Can you work these out from the model? Positions are in its coordinate system, mm. Give positions to 0.01 mm unless a question says otherwise; leave off trailing zeros. Order: outer loops, then holes, each group sorted by start corner. A loop starts at its lowest first (then second) coordinate and runs counter-clockwise, first axis right, second up. Notation, with made-up numbers: M 54,51 L 74,51 A32 ccw 74,79 Z; hole C 2.5,17.5 d6. An arc over 180 degrees is marked long. Answer as a JSON object with one key per item and string values.
```python
from build123d import *

# Parameters (mm, degrees)
EXTRUDE_1_DEPTH     = 8
SKETCH_3_R          = 3.1
SKETCH_3_R_2        = 1.6
CUT_EXTRUDE_1_DEPTH = 65.237839316
SKETCH_4_R          = 6.1
CUT_EXTRUDE_2_DEPTH = 65.237839316


with BuildPart() as part:
    # 草图1 → 凸台-拉伸1 (new body)
    with BuildSketch(Plane(origin=(0, 0, 0), x_dir=(1, 0, 0), z_dir=(0, 1, 0))):
        with BuildLine():
            Line((-50, -12.5), (50, -12.5))
            ThreePointArc((50, -12.5), (62.5, 0), (50, 12.5))
            Line((50, 12.5), (-50, 12.5))
            ThreePointArc((-50, 12.5), (-62.5, 0), (-50, -12.5))
        make_face()
    extrude(amount=EXTRUDE_1_DEPTH)

    # 草图3 → 切除-拉伸1 (cut, through all)
    with BuildSketch(Plane(origin=(0, 8, 0), x_dir=(1, 0, 0), z_dir=(0, 1, 0))):
        with Locations(Location((-50, 0, 0), (0, 0, 270))):
            Circle(SKETCH_3_R)
        with Locations(Location((50, 8, 0), (0, 0, 270))):
            Circle(SKETCH_3_R_2)
        with Locations(Location((58, 0, 0), (0, 0, 270))):
            Circle(SKETCH_3_R_2)
        with Locations(Location((50, -8, 0), (0, 0, 270))):
            Circle(SKETCH_3_R_2)
        with Locations(Location((42, 0, 0), (0, 0, 270))):
            Circle(SKETCH_3_R_2)
        with Locations(Location((50, 0, 0), (0, 0, 270))):
            Circle(SKETCH_3_R)
    extrude(amount=-CUT_EXTRUDE_1_DEPTH, mode=Mode.SUBTRACT)

    # 草图4 → 切除-拉伸2 (cut, through all)
    with BuildSketch(Plane(origin=(0, 8, 0), x_dir=(1, 0, 0), z_dir=(0, 1, 0))):
        with Locations(Location((-50, 0, 0), (0, 0, 270))):
            Circle(SKETCH_4_R)
    extrude(amount=-CUT_EXTRUDE_2_DEPTH, mode=Mode.SUBTRACT)


solid = part.part
```
1) I want a section at B-B on x = 42. Write out the boundary of the cut face in (y, z), and give its area (3 significant figures).
Results found:
{"outline": "M 0,-12.5 L 8,-12.5 L 8,-1.6 L 0,-1.6 Z; M 0,1.6 L 8,1.6 L 8,12.5 L 0,12.5 Z", "area": "174 mm²"}
2) I want a section at A-A on z = 0. Write out the boundary of the cut face in (x, y), and give its area (3 significant figures).
Results found:
{"outline": "M -62.5,0 L -56.1,0 L -56.1,8 L -62.5,8 Z; M -43.9,0 L 40.4,0 L 40.4,8 L -43.9,8 Z; M 43.6,0 L 46.9,0 L 46.9,8 L 43.6,8 Z; M 53.1,0 L 56.4,0 L 56.4,8 L 53.1,8 Z; M 59.6,0 L 62.5,0 L 62.5,8 L 59.6,8 Z", "area": "802 mm²"}
3) I need wall thicknesses on L1, parallel to X at y = 2.5, z = 0; L2, parallel to Z at x = -50.5, y = 1; L3, parallel to X at y = 6.5, z = -1.75. Which ranges of each line are inside material? Lowest first, please.
Results found:
{"L1": "x = -62.5 to -56.1, -43.9 to 40.4, 43.6 to 46.9, 53.1 to 56.4, 59.6 to 62.5", "L2": "z = -12.49 to -6.08, 6.08 to 12.49", "L3": "x = -62.38 to -55.84, -44.16 to 47.44, 52.56 to 62.38"}
4) I want a section at D-D on z = -8. Write out the boundary of the cut face in (x, y).
Results found:
{"outline": "M -59.6,0 L 48.4,0 L 48.4,8 L -59.6,8 Z; M 51.6,0 L 59.6,0 L 59.6,8 L 51.6,8 Z"}
5) Thinking about a two-plate mould opening in X: for faces 1 (the face through (-1, 0, 0)), 2 (the face through (-44.856, 4.056, 3.279)), 3 (the face through (-62.497, 3.944, -0.275)), which applies, pulls with the +X half, pulls with the -X half, needs draft (parallel to the pull), parting line crosses it, or undercut?
Results found:
{"face 1": "needs draft", "face 2": "undercut", "face 3": "pulls with the -X half"}
6) I want a section at C-C on y = 2.25. Write out the boundary of the cut face in (x, z).
Results found:
{"outline": "M -50,-12.5 L 50,-12.5 A12.5 ccw 50,12.5 L -50,12.5 A12.5 ccw Z; hole C -50,0 d12.2; hole C 42,0 d3.2; hole C 50,0 d6.2; hole C 50,-8 d3.2; hole C 50,8 d3.2; hole C 58,0 d3.2"}
7) I'm going to push flat-ended pins straight in: pin 1 Ø7 at (x, z) = (50, 0) entering from +Y; pin 2 Ø1.5 at (y, z) = (5, -5) entering from +X. Where does each tip first touch, or does it pass through?
Results found:
{"pin 1": "stops at y = 8", "pin 2": "stops at x = 61.76"}
